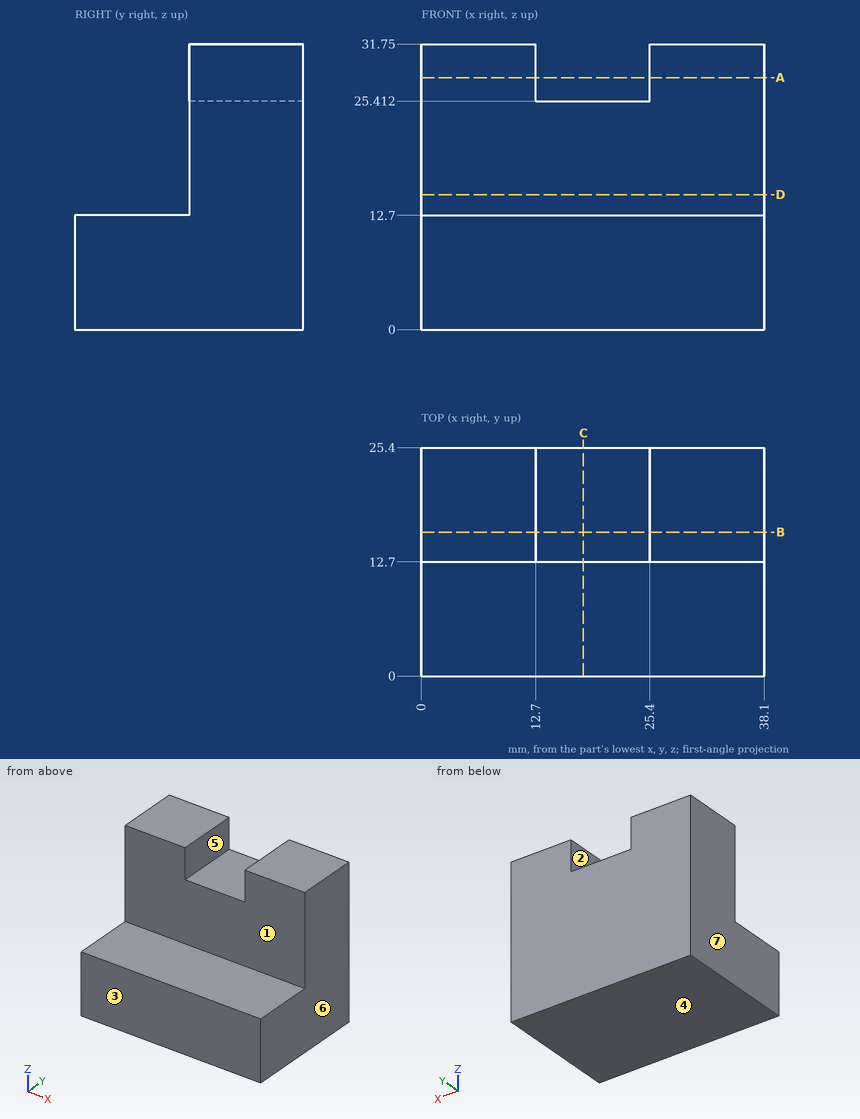
Source: three-view drawing plus pictorial views. Frame: mm from the lowest corner of the part. A direction names the side the tool comes from. Give positions to 0.01 mm unless a question says otherwise; leave off trailing zeros. Write each loop counter-clockwise with the first axis right and the second up, starting at its lowest first coordinate (ties: lowest second). Pieces come first, ordered by that corner, then holes. Notation, with made-up numbers: (64, 79.5) -> (68, 79.5) arc R13 ccw to (68, 102.5) -> close; hole circle Ø7 at (69.25, 9.5). An arc over 180 degrees is marked (long way). Answer in a Markdown table with one row per item.
(1) Section query D-D on z = 15. Return loops of the section in (x, y), then the cut area to 3 significant figures.
Answers below:
| item | result |
|---|---|
| outline | (0, 12.7) -> (38.1, 12.7) -> (38.1, 25.4) -> (0, 25.4) -> close |
| area | 484 mm^2 |
(2) Set-up query: the marked faces 1, 2 and 3. Return all of +Z, -Z, +X, -X, +Y, -Y with unobstructed straight access to the full face (end or side cutting, diameter ignored); none if empty.
Answers below:
| item | result |
|---|---|
| face 1 | +Z, +X, -X, -Y |
| face 2 | +Z, +Y, -Y |
| face 3 | +Z, -Z, +X, -X, -Y |
(3) Section query A-A on z = 28. Return loops of the section in (x, y), then the cut area to 3 significant figures.
Answers below:
| item | result |
|---|---|
| outline | (0, 12.7) -> (12.7, 12.7) -> (12.7, 25.4) -> (0, 25.4) -> close; (25.4, 12.7) -> (38.1, 12.7) -> (38.1, 25.4) -> (25.4, 25.4) -> close |
| area | 323 mm^2 |
(4) Section query B-B on y = 16. Return loops of the section in (x, z).
Answers below:
| item | result |
|---|---|
| outline | (0, 0) -> (38.1, 0) -> (38.1, 31.75) -> (25.4, 31.75) -> (25.4, 25.41) -> (12.7, 25.41) -> (12.7, 31.75) -> (0, 31.75) -> close |
(5) Ray query, line 1 along X through (y, z) = (14.25, 26); line 2 along Y through (x, z) = (10.5, 24.5); line 3 along Z through (x, y) = (20, 23.5). Return the intervals inside material, ascending. Write a range as [from, to].
Answers below:
| item | result |
|---|---|
| line 1 | [0, 12.7], [25.4, 38.1] |
| line 2 | [12.7, 25.4] |
| line 3 | [0, 25.41] |
(6) Draft query along X for the marked faces 4, 5, 6 and 7. Return one class per face: +X half, -X half, draft (parallel to the pull), parting line (faces both ways), or undercut.
Answers below:
| item | result |
|---|---|
| face 4 | draft |
| face 5 | undercut |
| face 6 | +X half |
| face 7 | -X half |
(7) Section query C-C on x = 18. Return loops of the section in (y, z).
Answers below:
| item | result |
|---|---|
| outline | (0, 0) -> (25.4, 0) -> (25.4, 25.41) -> (12.7, 25.41) -> (12.7, 12.7) -> (0, 12.7) -> close |
